Drawing for the job (mm, zero at the part's lowest x, y, z). Round coordinates to 2 decimals unless told otherwise and drop trailing zeros. Write each loop counter-clockwise with the first axis right and the second up, starting at its lowest first coordinate (ties: lowest second). Pieces come first, ordered by that corner, then holes.
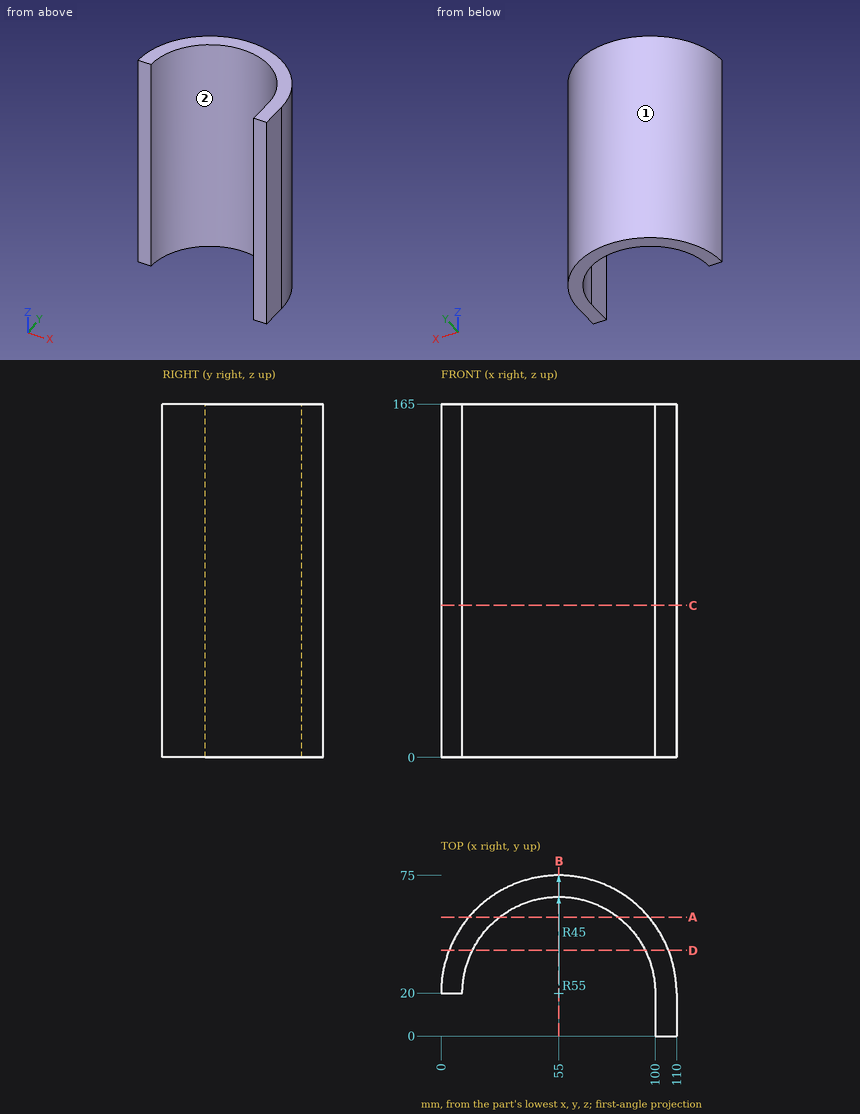
1) Cut at D-D on y = 40. List the corners of the cut face in (x, z), and give its area (3 significant figures).
2) Cut at B-B on x = 55. List the corners of the cut face in (y, z).
3) Pull direction X, two halves, no side cores. Call the marked faces 1 and 2: released by +X, released by -X, zero draft, split by the parting line, or undercut.
4) Cut at C-C on z = 71. List the corners of the cut face in (x, y), and give its area (3 significant figures).
5) Wall check: probe 1 along X at (y, z) = (39, 106); probe 2 along X at (y, z) = (52.5, 24.5); probe 3 along X at (y, z) = (18, 158.5). Give the ranges that are in metal, low to high.
6) Cut at A-A on y = 55.5. List the corners of the cut face in (x, z), and give its area (3 significant figures).
7) Flat gauge pins, fed straight in: pin 1 Ø4 at (x, z) = (89.5, 124.5) entering from +Y; pin 2 Ø1.5 at (x, z) = (18, 44.5) entering from +Y; pin 3 Ø4 at (y, z) = (12.5, 47) entering from -X. Where does each tip first touch, or does it go through?
Result sheet:
1. outline: (3.77, 0) - (14.69, 0) - (14.69, 165) - (3.77, 165) - close; (95.31, 0) - (106.23, 0) - (106.23, 165) - (95.31, 165) - close
1. area: 3,600 mm2
2. outline: (65, 0) - (75, 0) - (75, 165) - (65, 165) - close
3. face 1: split by the parting line
3. face 2: undercut
4. outline: (0, 20) - (10, 20) arc R45 cw to (100, 20) - (100, 0) - (110, 0) - (110, 20) arc R55 ccw to start
4. area: 1,770 mm2
5. probe 1: x = 3.39 to 14.21, 95.79 to 106.61
5. probe 2: x = 10.63 to 23.88, 86.12 to 99.37
5. probe 3: x = 100 to 110
6. outline: (12.99, 0) - (27.35, 0) - (27.35, 165) - (12.99, 165) - close; (82.65, 0) - (97.01, 0) - (97.01, 165) - (82.65, 165) - close
6. area: 4,740 mm2
7. pin 1: stops at y = 64.37
7. pin 2: stops at y = 61.36
7. pin 3: stops at x = 100
